Part model, mm, in its own coordinate system. A direction names the side the tool comes from. Round coordinates to 2 decimals unless told otherwise and drop trailing zeros. Write each loop counter-clockwise with the first axis right and the second up, starting at its lowest first coordinate (ties: lowest second). Pieces come first, ordered by that corner, then holes. Notation, with made-up numbers: M 61,-9 L 83,-9 A10 cw 83,10 Z; hole C 73.25,-6 d8. An arc over 180 degrees is marked long. Answer as a JSON object with one key per item and string values. Group by question number.
1. Which spindle directions (+Z, -Z, +X, -X, +Y, -Y) get a long thin tool onto all of the face, cutting with end or side? Do faces 1 (the face through (32, 23, 0)), 2 (the face through (42.48, 9.96, 0.99)). Say none if no direction does.
2. Drop a flat-ended pin along its axis: pin 1 (4 mm diameter, centred on x = 3, y = 42, fed in from +Z). Give the stop position or say it passes through.
3. Two-plate mould, pull along Y, no slides. Class faces 3 (the face through (15.12, 35.04, 0.99)), 4 (the face through (0, 22, 1)), 5 (the face through (32, 0, 1)): +Y half, -Y half, draft (parallel to the pull), parting line (faces both ways), or undercut.
4. Band-saw the part on B-B, the plane y = 42. Write the cut outline in (x, z).
5. Band-saw the part on A-A, the plane x = 3. Write the cut outline in (y, z), plus the area to 3 significant figures.
6. Drill centre lines: line 1 (Y direction, x = 3, z = 1.05); line 2 (Y direction, x = 20, z = 0.6); line 3 (X direction, y = 9, z = 0.4). Where is each one in solid material? Low to high. Write a range as from..to.
7. Band-saw the part on D-D, the plane y = 35. Write the cut outline in (x, z).
8. Band-saw the part on C-C, the plane z = 1. Write the cut outline in (x, y), plus the area to 3 significant figures.
from build123d import *

# Parameters (mm, degrees)
SKETCH_W  = 65
SKETCH_H  = 45
SKETCH_R  = 1.7
PAD_DEPTH = 2


with BuildPart() as part:
    # Sketch → Pad (new body)
    with BuildSketch(Plane.XY):
        with Locations((32.5, 22.5)):
            Rectangle(SKETCH_W, SKETCH_H)
        with Locations((3, 42)):
            Circle(SKETCH_R, mode=Mode.SUBTRACT)
        with Locations((62, 42)):
            Circle(SKETCH_R, mode=Mode.SUBTRACT)
        with Locations((3, 3)):
            Circle(SKETCH_R, mode=Mode.SUBTRACT)
        with Locations((62, 3)):
            Circle(SKETCH_R, mode=Mode.SUBTRACT)
        with BuildLine():
            ThreePointArc((17.118392, 37), (15.118392, 35), (17.118392, 33))
            Line((17.118392, 33), (40.47904, 33))
            ThreePointArc((40.47904, 33), (42.47904, 35), (40.47904, 37))
            Line((17.118392, 37), (40.47904, 37))
        make_face(mode=Mode.SUBTRACT)
        with BuildLine():
            ThreePointArc((17.118392, 12), (15.118392, 10), (17.118392, 8))
            Line((17.118392, 8), (40.47904, 8))
            ThreePointArc((40.47904, 8), (42.47904, 10), (40.47904, 12))
            Line((17.118392, 12), (40.47904, 12))
        make_face(mode=Mode.SUBTRACT)
    extrude(amount=PAD_DEPTH)


solid = part.part
Worked answers:
{
 "1": {"face 1": "-Z, +X, -X, +Y, -Y", "face 2": "+Z, -Z"},
 "2": {"pin 1": "stops at z = 2"},
 "3": {"face 3": "undercut", "face 4": "draft", "face 5": "-Y half"},
 "4": {"outline": "M 0,0 L 1.3,0 L 1.3,2 L 0,2 Z; M 4.7,0 L 60.3,0 L 60.3,2 L 4.7,2 Z; M 63.7,0 L 65,0 L 65,2 L 63.7,2 Z"},
 "5": {"outline": "M 0,0 L 1.3,0 L 1.3,2 L 0,2 Z; M 4.7,0 L 40.3,0 L 40.3,2 L 4.7,2 Z; M 43.7,0 L 45,0 L 45,2 L 43.7,2 Z", "area": "76.4 mm^2"},
 "6": {"line 1": "y = 0..1.3, 4.7..40.3, 43.7..45", "line 2": "y = 0..8, 12..33, 37..45", "line 3": "x = 0..15.39, 42.21..65"},
 "7": {"outline": "M 0,0 L 15.12,0 L 15.12,2 L 0,2 Z; M 42.48,0 L 65,0 L 65,2 L 42.48,2 Z"},
 "8": {"outline": "M 0,0 L 65,0 L 65,45 L 0,45 Z; hole C 3,3 d3.4; hole C 3,42 d3.4; hole M 17.12,8 L 40.48,8 A2 ccw 40.48,12 L 17.12,12 A2 ccw Z; hole M 17.12,33 L 40.48,33 A2 ccw 40.48,37 L 17.12,37 A2 ccw Z; hole C 62,3 d3.4; hole C 62,42 d3.4", "area": "2,680 mm^2"}
}
